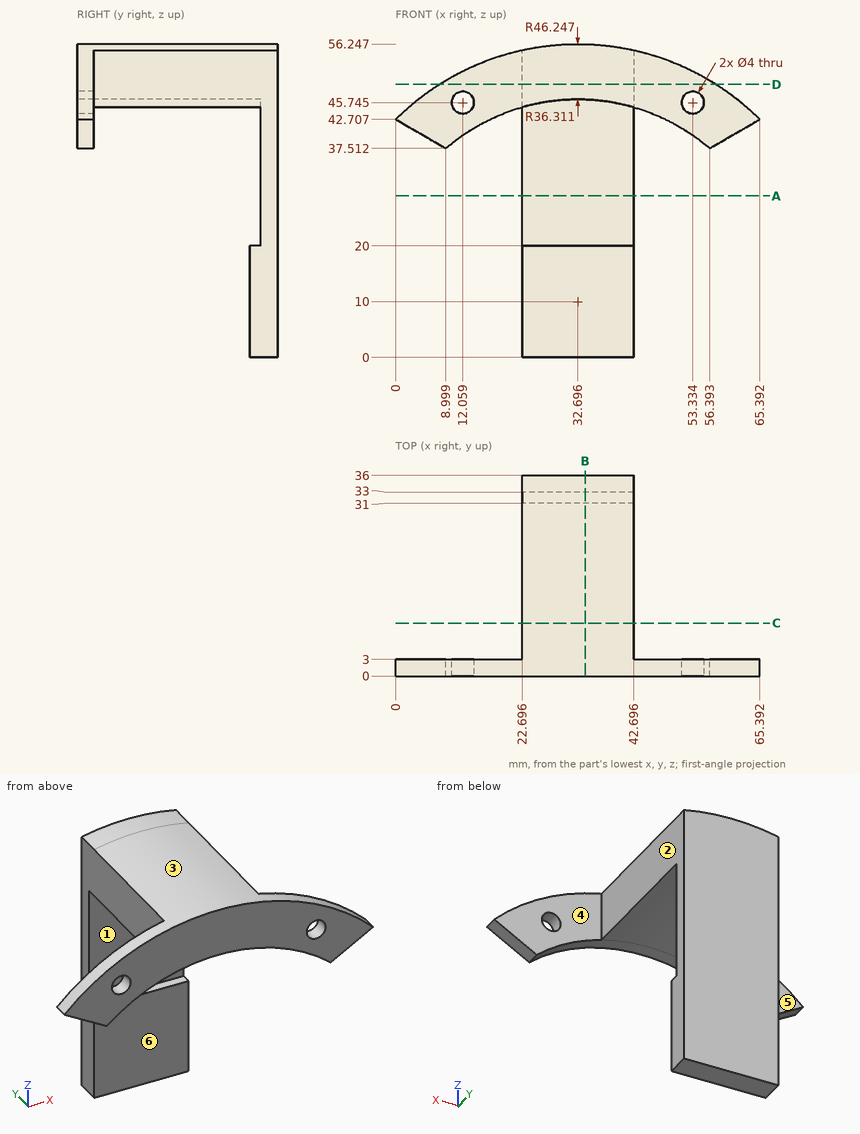
Source: three-view drawing plus pictorial views. Frame: mm from the lowest corner of the part. A direction names the side the tool comes from. Give positions to 0.01 mm unless a question says otherwise; leave off trailing zeros. Write each loop counter-clockwise with the first axis right and the second up, starting at its lowest first coordinate (ties: lowest second). Pieces come first, ordered by that corner, then holes. Notation, with made-up numbers: M 5,68.25 L 18,68.25 A18 ccw 18,84.25 Z; hole C 8,-10 d7. An arc over 180 degrees is marked long. Use one line per item in the form item = value.
1. Reachability of the marked faces 4, 5 and 6 from +Z, -Z, +X, -X, +Y, -Y: full face, straight path, thin tool, end or side. Return the list, or none.
Outcome:
face_4 = +Z, -Z, +X, +Y
face_5 = +Z, -Z, -X, +Y
face_6 = -Z, +X, -X, -Y
2. Cut plane D-D on z = 49. Return loops of the section in (x, y) (1 decimal).
Outcome:
outline = M 7.8,0 L 57.6,0 L 57.6,3 L 42.7,3 L 42.7,36 L 22.7,36 L 22.7,3 L 7.8,3 Z
3. Cut plane B-B on x = 34. Return loops of the section in (y, z), and give its area (3 significant figures).
Outcome:
outline = M 0,46.29 L 33,46.29 L 33,20 L 31,20 L 31,0 L 36,0 L 36,56.23 L 0,56.23 Z
area = 537 mm²
4. Mould query, pull axis Z, two halves, no side actions, for the marked faces 1, 2 and 3. Classes: released by +Z, released by -Z, zero draft, split by the parting line, or undercut.
Outcome:
face_1 = undercut
face_2 = zero draft
face_3 = released by +Z
5. First-contact query: P1, Ø6, axis at y = 20.5, z = 47, coming from the -X side; P2, Ø3, axis at y = 30, z = 15.5, coming from the +X side; P3, Ø10, axis at y = 20, z = 37.5, coming from the +X side; P4, Ø0.6, axis at x = 36, y = 31.5, coming from the +Z side. Flat tips, straight axial feed; report the tip coordinate or a pass-through.
Outcome:
P1 = 22.7
P2 = 42.7
P3 = through
P4 = 56.15
6. Cut plane C-C on y = 9.5. Return loops of the section in (x, z) (1 decimal), and give its area (3 significant figures).
Outcome:
outline = M 22.7,44.9 A36.3 cw 42.7,44.9 L 42.7,55.2 A46.2 ccw 22.7,55.2 Z
area = 201 mm²
7. Ray query, L1, parallel to Y at x = 53, z = 41.5; L2, parallel to Y at x = 41, z = 35.5; L3, parallel to X at y = 14, z = 47 (1 decimal). Return the intervals inside material, ascending.
Outcome:
L1 = 0 to 3
L2 = 33 to 36
L3 = 22.7 to 42.7
8. Cut plane A-A on z = 29. Return loops of the section in (x, y) (1 decimal).
Outcome:
outline = M 22.7,33 L 42.7,33 L 42.7,36 L 22.7,36 Z
